The listing builds one solid part. Answer for the finished solid, in the listing's coordinates (mm). Face numbers are marked on the shaded views. A direction names the side the tool comes from. Coordinates: 2 decimals unless noted, no trailing zeros. Order: outer loops, then holes, each group sorted by start corner. A loop starts at its lowest first (then second) coordinate and runs counter-clockwise, first axis right, second up. Notation, with made-up numbers: (-31, 65) -> (-3, 65) arc R24 ccw to (-3, 103) -> close; hole circle Ø5 at (-3, 25). An arc over 180 degrees is marked (long way). Return JSON: item names as keys, results as strings.
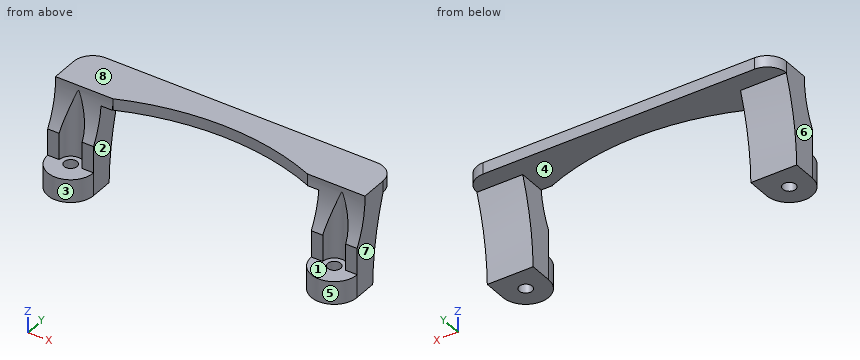
from build123d import *

# Parameters (mm, degrees)
IZIM1_R                       = 6
IZIM1_R_2                     = 1.7
Y_KSEKLIK_EKSTR_ZYON1_DEPTH   = 22
Y_KSEKLIK_EKSTR_ZYON1_2_DEPTH = 22
IZIM2_R                       = 1.7
Y_KSEKLIK_EKSTR_ZYON2_DEPTH   = 3
RADYUS2_R                     = 5
IZIM4_R                       = 1.6
KES_EKSTR_ZYON1_DEPTH         = 10
Y_KSEKLIK_EKSTR_ZYON5_DEPTH   = 12
Y_KSEKLIK_EKSTR_ZYON6_DEPTH   = 12
KES_EKSTR_ZYON2_DEPTH         = 97
IZIM10_W                      = 6.92309327
IZIM10_H                      = 6.61748972
KES_EKSTR_ZYON3_DEPTH         = 97
IZIM11_R                      = 3
KES_EKSTR_ZYON4_DEPTH         = 97
IZIM12_R                      = 1.6
Y_KSEKLIK_EKSTR_ZYON8_DEPTH   = 10
IZIM13_R                      = 1.7
KES_EKSTR_ZYON5_DEPTH         = 10
KES_EKSTR_ZYON6_DEPTH         = 10


with BuildPart() as part:
    # izim1 → Y_kseklik-Ekstr_zyon1 (new body)
    with BuildSketch(Plane.XY):
        with Locations((34.5, 0)):
            Circle(IZIM1_R)
        with Locations((34.5, 0)):
            Circle(IZIM1_R_2, mode=Mode.SUBTRACT)
    extrude(amount=Y_KSEKLIK_EKSTR_ZYON1_DEPTH)



with BuildPart() as body_2:
    # izim1 → Y_kseklik-Ekstr_zyon1 2 (new body)
    with BuildSketch(Plane.XY):
        with Locations((-34.5, 0)):
            Circle(IZIM1_R)
        with Locations((-34.5, 0)):
            Circle(IZIM1_R_2, mode=Mode.SUBTRACT)
    extrude(amount=Y_KSEKLIK_EKSTR_ZYON1_2_DEPTH)


with BuildPart() as part_1:
    add(part.part)

    add(body_2.part)  # Y_kseklik-Ekstr_zyon2 merges body 2
    # izim2 → Y_kseklik-Ekstr_zyon2 (add)
    with BuildSketch(Plane.XY.offset(22)):
        with BuildLine():
            Line((-40.5, 0), (-40.5, 10))
            Line((-40.5, 10), (-40.5, 15))
            Line((-40.5, 15), (40.5, 15))
            Line((40.5, 15), (40.5, 10))
            Line((40.5, 10), (40.5, 0))
            ThreePointArc((40.5, 0), (37.400947284, -5.252095282), (31.305165048, -5.078683848))
            ThreePointArc((31.305165048, -5.078683848), (23.833029749, -2.135860906), (16.017952, -0.287193122))
            ThreePointArc((16.017952, -0.287193122), (8.530102356, 4.184082865), (0, 6))
            ThreePointArc((0, 6), (-8.530102356, 4.184082865), (-16.017952, -0.287193122))
            ThreePointArc((-16.017952, -0.287193122), (-23.833029749, -2.135860906), (-31.305165048, -5.078683848))
            ThreePointArc((-31.305165048, -5.078683848), (-37.400947284, -5.252095282), (-40.5, 0))
        make_face()
        with Locations((-34.5, 0)):
            Circle(IZIM2_R, mode=Mode.SUBTRACT)
        with Locations((34.5, 0)):
            Circle(IZIM2_R, mode=Mode.SUBTRACT)
    extrude(amount=Y_KSEKLIK_EKSTR_ZYON2_DEPTH)

    # Radyus2
    radyus2_edges = [part_1.edges().sort_by_distance(p)[0] for p in [
        (40.5, 15, 23.5),
        (-40.5, 15, 23.5),
    ]]
    fillet(radyus2_edges, radius=RADYUS2_R)

    # izim4 → Kes-Ekstr_zyon1 (cut)
    with BuildSketch(Plane.XY.offset(25)):
        with Locations((-35, 5)):
            Circle(IZIM4_R)
        with Locations((35, 5)):
            Circle(IZIM4_R)
    extrude(amount=-KES_EKSTR_ZYON1_DEPTH, mode=Mode.SUBTRACT)

    # izim5 → Y_kseklik-Ekstr_zyon5 (add)
    with BuildSketch(Plane.ZY.offset(40.5)):
        with BuildLine():
            Line((0, 6), (0, 0))
            Line((0, 0), (22, 0))
            Line((22, 0), (22, 10))
            ThreePointArc((22, 10), (11.160931836, 7.114874904), (0, 6))
        make_face()
    extrude(amount=-Y_KSEKLIK_EKSTR_ZYON5_DEPTH)

    # izim6 → Y_kseklik-Ekstr_zyon6 (add)
    with BuildSketch(Plane(origin=(40.5, 0, 0), x_dir=(0, 0, -1), z_dir=(1, 0, 0))):
        with BuildLine():
            Line((-22, 0), (-22, 10))
            ThreePointArc((-22, 10), (-11.160931836, 7.114874904), (0, 6))
            Line((0, 6), (0, 0))
            Line((0, 0), (-22, 0))
        make_face()
    extrude(amount=-Y_KSEKLIK_EKSTR_ZYON6_DEPTH)

    # izim9 → Kes-Ekstr_zyon2 (cut)
    with BuildSketch(Plane.ZY.offset(40.5)):
        with BuildLine():
            Line((25, 3), (25, -6.889643691))
            Line((25, -6.889643691), (6, -6))
            ThreePointArc((6, -6), (14.421146183, 0.77758028), (25, 3))
        make_face()
    extrude(amount=-KES_EKSTR_ZYON2_DEPTH, mode=Mode.SUBTRACT)

    # izim10 → Kes-Ekstr_zyon3 (cut)
    with BuildSketch(Plane.ZY.offset(40.5)):
        with Locations((9.461563543, -3.30874486)):
            Rectangle(IZIM10_W, IZIM10_H)
    extrude(amount=-KES_EKSTR_ZYON3_DEPTH, mode=Mode.SUBTRACT)

    # izim11 → Kes-Ekstr_zyon4 (cut)
    with BuildSketch(Plane.XY.offset(6.000016908)):
        with Locations((-34.5, 0)):
            Circle(IZIM11_R)
        with Locations((34.5, 0)):
            Circle(IZIM11_R)
    extrude(amount=KES_EKSTR_ZYON4_DEPTH, mode=Mode.SUBTRACT)

    # izim12 → Y_kseklik-Ekstr_zyon8 (add)
    with BuildSketch(Plane.XY.offset(25)):
        with Locations((-35, 5)):
            Circle(IZIM12_R)
        with Locations((35, 5)):
            Circle(IZIM12_R)
    extrude(amount=-Y_KSEKLIK_EKSTR_ZYON8_DEPTH)

    # izim13 → Kes-Ekstr_zyon5 (cut)
    with BuildSketch(Plane(origin=(0, 0, 0), x_dir=(-1, 0, 0), z_dir=(0, 0, -1))):
        with Locations((34.5, 0)):
            Circle(IZIM13_R)
        with Locations((-34.5, 0)):
            Circle(IZIM13_R)
    extrude(amount=-KES_EKSTR_ZYON5_DEPTH, mode=Mode.SUBTRACT)

    # izim15 → Kes-Ekstr_zyon6 (cut)
    with BuildSketch(Plane.XY.offset(25)):
        with BuildLine():
            Line((-25.5, 3), (-25.5, -6.328988838))
            Line((-25.5, -6.328988838), (21.982441761, -11.682646241))
            Line((21.982441761, -11.682646241), (25.5, 3))
            ThreePointArc((25.5, 3), (0, 8.028595904), (-25.5, 3))
        make_face()
    extrude(amount=-KES_EKSTR_ZYON6_DEPTH, mode=Mode.SUBTRACT)


solid = part_1.part
1. The part is cut by section D-D on y = 12.75. Give the vertices of the cut face in (x, z), and give its area (3 significant figures).
Answer block:
{"outline": "(-39.68, 22) -> (39.68, 22) -> (39.68, 25) -> (-39.68, 25) -> close", "area": "238 mm2"}
2. For the marked faces 1, 2, 3 and 4, determine the directions among +Z, -Z, +X, -X, +Y, -Y from which every point of the face is accessible in a straight line to the end or side of a thin tool.
Answer block:
{"face 1": "+Z, -Y", "face 2": "-Z, +Y, -Y", "face 3": "+Z, -Z, -Y", "face 4": "-Z, +Y"}
3. The part is cut by section A-A on z = 3. Give the vertices of the cut face in (x, y), and give its area (3 significant figures).
Answer block:
{"outline": "(-40.5, 0) arc R6 ccw to (-28.5, 0) -> (-28.5, 6.12) -> (-40.5, 6.12) -> close; (28.5, 0) arc R6 ccw to (40.5, 0) -> (40.5, 6.12) -> (28.5, 6.12) -> close; hole circle Ø3.4 at (-34.5, 0); hole circle Ø3.4 at (34.5, 0)", "area": "242 mm2"}
4. Consider line 1 (X direction, y = 0, z = 3); line 2 (X direction, y = 5, z = 4.25); line 3 (Z direction, x = -21.5, y = 11.5). Determine where each line is inside the solid, lowest interval first. Write a range as from..to.
Answer block:
{"line 1": "x = -40.5..-36.2, -32.8..-28.5, 28.5..32.8, 36.2..40.5", "line 2": "x = -40.5..-28.5, 28.5..40.5", "line 3": "z = 22..25"}
5. The part is cut by section C-C on x = -21. Give the vertices of the cut face in (y, z), and give its area (3 significant figures).
Answer block:
{"outline": "(4.66, 22) -> (15, 22) -> (15, 25) -> (4.66, 25) -> close", "area": "31.0 mm2"}
6. Determine the mould class of the marked faces 5, 6, 7 and 8 for opening direction X: pulls with the +X half, pulls with the -X half, needs draft (parallel to the pull), parting line crosses it, or undercut.
Answer block:
{"face 5": "undercut", "face 6": "pulls with the -X half", "face 7": "pulls with the +X half", "face 8": "needs draft"}
7. Each of these flat-tipped pins is pushed along its axis until it touches: pin 1 Ø2 at (x, y) = (24, 5.5) entering from -Z; pin 2 Ø3.5 at (x, z) = (-30.5, 10) entering from -Y; pin 3 Ø8 at (x, z) = (-25, 16) entering from -Y. Where does it stop, or does it pass through?
Answer block:
{"pin 1": "stops at z = 22", "pin 2": "stops at y = 0", "pin 3": "stops at y = 0.6"}
8. The part is cut by section B-B on z = 16.25. Give the vertices of the cut face in (x, y).
Answer block:
{"outline": "(-40.5, 1.55) -> (-37.07, 1.55) arc R3 cw to (-31.93, 1.55) -> (-28.5, 1.55) -> (-28.5, 8.24) -> (-40.5, 8.24) -> close; (28.5, 1.55) -> (31.93, 1.55) arc R3 cw to (37.07, 1.55) -> (40.5, 1.55) -> (40.5, 8.24) -> (28.5, 8.24) -> close"}
